```python
from build123d import *

# Parameters (mm, degrees)
SZKIC1_R                    = 6
DODANIE_WYCI_GNI_CIE1_DEPTH = 5
SZKIC2_R                    = 7.5
DODANIE_WYCI_GNI_CIE2_DEPTH = 10
SFAZOWANIE1_SIZE            = 2
SFAZOWANIE1_SIZE2           = 1.154700538
ZAOKR_GLENIE1_R             = 5


with BuildPart() as part:
    # Szkic1 → Dodanie-wyciągnięcie1 (new body)
    with BuildSketch(Plane.XY):
        Circle(SZKIC1_R)
    extrude(amount=DODANIE_WYCI_GNI_CIE1_DEPTH)

    # Szkic2 → Dodanie-wyciągnięcie2 (add)
    with BuildSketch(Plane.XY):
        Circle(SZKIC2_R)
    extrude(amount=-DODANIE_WYCI_GNI_CIE2_DEPTH)

    # Sfazowanie1
    sfazowanie1_edges = [part.edges().sort_by_distance(p)[0] for p in [
        (-6, 0, 5),
    ]]
    sfazowanie1_side = [part.faces().sort_by_distance(p)[0] for p in [
        (-6, 0, 2.5),
    ]]
    chamfer(sfazowanie1_edges, length=SFAZOWANIE1_SIZE, length2=SFAZOWANIE1_SIZE2, reference=sfazowanie1_side[0])

    # Zaokrąglenie1
    # the kernel refuses this fillet: 5 mm, written as the material it takes off along each edge
    with BuildSketch(Plane(origin=(0, 0, 0), x_dir=(1, 0, 0), z_dir=(0, -1, 0))) as zaokr_glenie1_piece_1:
        with BuildLine():
            CenterArc((2.5, -3.570714214), ZAOKR_GLENIE1_R, 0, 45.572995999)
            Line((7.5, -3.570714214), (7.6, -3.570714214))
            Line((7.6, -3.570714214), (7.6, 0))
            Line((7.6, 0), (7.5, 0.1))
            ThreePointArc((7.5, 0.1), (6.75, 0.1), (6.07, 0.071414284))
            Line((6.07, 0.071414284), (6, 0))
        make_face()
    revolve(axis=Axis((0, 0, 0), (0, 0, 1)), mode=Mode.SUBTRACT)


solid = part.part
```
Check sheet for the modelled part. Datum: model origin and axes. Units: mm. A direction names the side the tool comes from. Coordinates: 2 decimals unless noted, no trailing zeros. Write each loop counter-clockwise with the first axis right and the second up, starting at its lowest first coordinate (ties: lowest second). Pieces come first, ordered by that corner, then holes. Notation, with made-up numbers: M 83.5,74 L 90.5,74 A20 ccw 90.5,93 Z; hole C 6,25 d6. An arc over 180 degrees is marked long. Write item = value, one per line. Start each with the question number.
1. Go/stop test with flat-tipped pins: pin 1 (1.5 mm diameter, centred on y = -1, z = -6, fed in from +X); pin 2 (1 mm diameter, centred on x = 5, z = -4.5, fed in from +Y); pin 3 (1 mm diameter, centred on x = -5.5, z = -6.5, fed in from -Y). Record where each tip stops, or that it passes through.
2. Thickness scan on probe 1 along Y at (x, z) = (4.5, -8.25); probe 2 along X at (y, z) = (-4, -0.5); probe 3 along X at (y, z) = (-1.5, -7). Record the ranges inside material, lowest first.
3. Sectioned sample at A-A (z = -4). Record the cut outline in (x, y).
4. Tool access check on faces 1 (the cylindrical face through (-6, 0, 1)), 2 (the flat face through (0, 0, 5)). Record the directions out of +Z, -Z, +X, -X, +Y, -Y that give a thin tool (end or side, any length) a straight path to the whole face; none if there is none.
5. Sectioned sample at B-B (z = 1). Record the cut outline in (x, y).
The answers:
q1.pin_1 = 7.5
q1.pin_2 = 6
q1.pin_3 = -5.59
q2.probe_1 = -6 to 6
q2.probe_2 = -5.05 to 5.05
q2.probe_3 = -7.35 to 7.35
q3.outline = C 0,0 d15
q4.face_1 = +Z
q4.face_2 = +Z, +X, -X, +Y, -Y
q5.outline = C 0,0 d12
